Part model, mm, in its own coordinate system. A direction names the side the tool comes from. Round coordinates to 2 decimals unless told otherwise and drop trailing zeros. Write each loop counter-clockwise with the first axis right and the second up, starting at its lowest first coordinate (ties: lowest second). Pieces come first, ordered by that corner, then holes.
1) Pull direction Y, two halves, no side cores. Call faces 1 (the conical face through (-6.06, 0.45, 1.06)), 2 (the cylindrical face through (-6.57, 8.39, 1.31)), 3 (the flat face through (-0.2, 5.7, 0)): +Y half, -Y half, draft (parallel to the pull), parting line (faces both ways), or undercut.
2) Saw through at D-D on y = -4. Write the cut outline in (x, z), and give its area (3 significant figures).
3) Flat gauge pin, fed straight in: pin 1 (2.5 mm diameter, centred on x = 0, y = -7.5, fed in from +Z). Where does the tip first touch, or does it go through?
4) Saw through at A-A on x = 0. Write the cut outline in (y, z), and give its area (3 significant figures).
5) Drill centre lines: L1, parallel to Y at x = 0, z = 0.4; L2, parallel to Y at x = 3.25, z = 1.1; L3, parallel to Y at x = -0.5, z = 0.4. Where is each one in solid material? Low to high.
6) Saw through at C-C on z = 0.55. Count the separate pieces of the cut face and the enclosed holes in it, and give its area (3 significant figures).
7) Which spindle directions (+Z, -Z, +X, -X, +Y, -Y) get a long thin tool onto all of the face, cutting with end or side? Do faces 4 (the flat face through (0, 4.5, 1)), 5 (the conical face through (-0.327, -8.971, 1.056)). Say none if no direction does.
```python
from build123d import *

# Parameters (mm, degrees)
SKETCH_1_W      = 25
SKETCH_1_H      = 25
SKETCH_1_R      = 1.4
SKETCH_1_R_2    = 1.45
SKETCH_1_W_2    = 9
SKETCH_1_H_2    = 9
EXTRUDE_1_DEPTH = 2.65
CHAMFER_1_SIZE  = 1.7
FILLET_1_R      = 1


with BuildPart() as part:
    # 草图1 → 凸台-拉伸1 (new body)
    with BuildSketch(Plane.XY):
        Rectangle(SKETCH_1_W, SKETCH_1_H)
        with Locations((0, 7.5)):
            Circle(SKETCH_1_R, mode=Mode.SUBTRACT)
        with Locations((7.5, 0)):
            Circle(SKETCH_1_R, mode=Mode.SUBTRACT)
        with Locations((0, -7.5)):
            Circle(SKETCH_1_R, mode=Mode.SUBTRACT)
        with Locations((-7.5, 0)):
            Circle(SKETCH_1_R, mode=Mode.SUBTRACT)
        with Locations((7.954951288, 7.954951288)):
            Circle(SKETCH_1_R_2, mode=Mode.SUBTRACT)
        with Locations((7.954951288, -7.954951288)):
            Circle(SKETCH_1_R_2, mode=Mode.SUBTRACT)
        with Locations((-7.954951288, -7.954951288)):
            Circle(SKETCH_1_R_2, mode=Mode.SUBTRACT)
        with Locations((-7.954951288, 7.954951288)):
            Circle(SKETCH_1_R_2, mode=Mode.SUBTRACT)
        Rectangle(SKETCH_1_W_2, SKETCH_1_H_2, mode=Mode.SUBTRACT)
    extrude(amount=EXTRUDE_1_DEPTH)

    # 倒角1
    # the kernel refuses this chamfer: 1.7 mm, written as the material it takes off along each edge
    with BuildSketch(Plane(origin=(0, 7.5, 2.65), x_dir=(1, 0, 0), z_dir=(0, -1, 0))) as chamfer_1_piece_1:
        Polygon((1.4, -CHAMFER_1_SIZE), (1.4 + CHAMFER_1_SIZE, 0), (1.4, 0), align=None)
    revolve(axis=Axis((0, 7.5, 2.65), (0, 0, 1)), mode=Mode.SUBTRACT)
    with BuildSketch(Plane(origin=(7.5, 0, 2.65), x_dir=(1, 0, 0), z_dir=(0, -1, 0))) as chamfer_1_piece_2:
        Polygon((1.4, -CHAMFER_1_SIZE), (1.4 + CHAMFER_1_SIZE, 0), (1.4, 0), align=None)
    revolve(axis=Axis((7.5, 0, 2.65), (0, 0, 1)), mode=Mode.SUBTRACT)
    with BuildSketch(Plane(origin=(0, -7.5, 2.65), x_dir=(1, 0, 0), z_dir=(0, -1, 0))) as chamfer_1_piece_3:
        Polygon((1.4, -CHAMFER_1_SIZE), (1.4 + CHAMFER_1_SIZE, 0), (1.4, 0), align=None)
    revolve(axis=Axis((0, -7.5, 2.65), (0, 0, 1)), mode=Mode.SUBTRACT)
    with BuildSketch(Plane(origin=(-7.5, 0, 2.65), x_dir=(1, 0, 0), z_dir=(0, -1, 0))) as chamfer_1_piece_4:
        Polygon((1.4, -CHAMFER_1_SIZE), (1.4 + CHAMFER_1_SIZE, 0), (1.4, 0), align=None)
    revolve(axis=Axis((-7.5, 0, 2.65), (0, 0, 1)), mode=Mode.SUBTRACT)

    # 圆角1
    fillet_1_edges = [part.edges().sort_by_distance(p)[0] for p in [
        (4.5, -4.5, 1.325),
        (4.5, 4.5, 1.325),
        (-4.5, 4.5, 1.325),
        (-4.5, -4.5, 1.325),
    ]]
    fillet(fillet_1_edges, radius=FILLET_1_R)


solid = part.part
```
Completed:
1. face 1: undercut
1. face 2: undercut
1. face 3: draft
2. outline: (-12.5, 0) - (-4.37, 0) - (-4.37, 2.65) - (-12.5, 2.65) - close; (4.37, 0) - (12.5, 0) - (12.5, 2.65) - (4.37, 2.65) - close
2. area: 43.1 mm2
3. pin 1: passes through
4. outline: (-12.5, 0) - (-8.9, 0) - (-8.9, 0.95) - (-10.6, 2.65) - (-12.5, 2.65) - close; (-6.1, 0) - (-4.5, 0) - (-4.5, 2.55) - (-6.1, 0.95) - close; (4.5, 0) - (6.1, 0) - (6.1, 0.95) - (4.5, 2.55) - close; (8.9, 0) - (12.5, 0) - (12.5, 2.65) - (10.6, 2.65) - (8.9, 0.95) - close
4. area: 21.8 mm2
5. L1: y = -12.5 to -8.9, -6.1 to -4.5, 4.5 to 6.1, 8.9 to 12.5
5. L2: y = -12.5 to -4.5, 4.5 to 12.5
5. L3: y = -12.5 to -8.81, -6.19 to -4.5, 4.5 to 6.19, 8.81 to 12.5
6. separate pieces: 1
6. enclosed holes: 9
6. area: 494 mm2
7. face 4: +Z, -Z
7. face 5: +Z
